Geometry check sheet. Reference: the model listing, model coordinates, mm. A direction names the side the tool comes from. Round coordinates to 2 decimals unless told otherwise and drop trailing zeros. Loops run counter-clockwise (first coordinate to the right, second up) from the corner with the lowest first, then second, coordinate; pieces in that order, holes last. Notation, with made-up numbers: (67, 32.5) -> (95, 32.5) arc R23 cw to (95, 50.5) -> close; hole circle Ø4 at (78, 25.5). An arc over 180 degrees is marked (long way). Use one line per item in the form item = value.
from build123d import *

# Parameters (mm, degrees)
SKETCH_1_R      = 1.25
EXTRUDE_1_DEPTH = 2


with BuildPart() as part:
    # 草圖1 → 填料-伸長1 (new body)
    with BuildSketch(Plane.XY):
        with BuildLine():
            Line((18.048613933, -20.404186252), (23.048613933, -20.404186252))
            ThreePointArc((23.048613933, -20.404186252), (23.755720714, -20.111293033), (24.048613933, -19.404186252))
            Line((24.048613933, -19.404186252), (24.048613933, -15.404186252))
            Line((24.048613933, -15.404186252), (24.048613933, -2.404186252))
            ThreePointArc((24.048613933, -2.404186252), (23.755720714, -1.697079471), (23.048613933, -1.404186252))
            Line((23.048613933, -1.404186252), (-6.951386067, -1.404186252))
            ThreePointArc((-6.951386067, -1.404186252), (-7.658492848, -1.697079471), (-7.951386067, -2.404186252))
            Line((-7.951386067, -2.404186252), (-7.951386067, -15.404186252))
            Line((-7.951386067, -15.404186252), (-7.951386067, -19.404186252))
            ThreePointArc((-7.951386067, -19.404186252), (-7.658492848, -20.111293033), (-6.951386067, -20.404186252))
            Line((-6.951386067, -20.404186252), (-1.951386067, -20.404186252))
            ThreePointArc((-1.951386067, -20.404186252), (-1.244279286, -20.697079471), (-0.951386067, -21.404186252))
            Line((-0.951386067, -21.404186252), (-0.951386067, -60.404186252))
            ThreePointArc((-0.951386067, -60.404186252), (8.048613933, -69.404186252), (17.048613933, -60.404186252))
            Line((17.048613933, -60.404186252), (17.048613933, -21.404186252))
            ThreePointArc((17.048613933, -21.404186252), (17.341507152, -20.697079471), (18.048613933, -20.404186252))
        make_face()
        with Locations((8.048613933, -60.404186252)):
            Circle(SKETCH_1_R, mode=Mode.SUBTRACT)
        with Locations((-5.451386067, -17.904186252)):
            Circle(SKETCH_1_R, mode=Mode.SUBTRACT)
        with Locations((21.548613933, -17.904186252)):
            Circle(SKETCH_1_R, mode=Mode.SUBTRACT)
    extrude(amount=EXTRUDE_1_DEPTH)


solid = part.part
1. Material ranges on line 1 along Y through (x, z) = (-5.5, 1); line 2 along X through (y, z) = (-45.5, 0.6); line 3 along X through (y, z) = (-61.5, 0.1), recorded low to high.
Return value:
line_1 = -20.4 to -19.15, -16.66 to -1.4
line_2 = -0.95 to 17.05
line_3 = -0.88 to 7.45, 8.65 to 16.98
2. Mould release check, pull along X, two halves, no side actions. Record for faces 1 (the cylindrical face through (-5.722, -19.124, 0.986)), 2 (the cylindrical face through (7.85, -69.4, 0.99)), 3 (the flat face through (8, -27, 2)): released by +X, released by -X, zero draft, split by the parting line, or undercut.
Return value:
face_1 = undercut
face_2 = split by the parting line
face_3 = zero draft
3. Section check B-B (x = 21.5). Record the boundary of the cut face in (y, z), then the cut area to 3 significant figures.
Return value:
outline = (-20.4, 0) -> (-19.15, 0) -> (-19.15, 2) -> (-20.4, 2) -> close; (-16.66, 0) -> (-1.4, 0) -> (-1.4, 2) -> (-16.66, 2) -> close
area = 33.0 mm2
4. Section check D-D (x = -5). Record the boundary of the cut face in (y, z).
Return value:
outline = (-20.4, 0) -> (-19.07, 0) -> (-19.07, 2) -> (-20.4, 2) -> close; (-16.74, 0) -> (-1.4, 0) -> (-1.4, 2) -> (-16.74, 2) -> close
5. Section check A-A (z = 1). Record the boundary of the cut face in (x, y), then the cut area to 3 significant figures.
Return value:
outline = (-7.95, -19.4) arc R1 ccw to (-6.95, -20.4) -> (-1.95, -20.4) arc R1 cw to (-0.95, -21.4) -> (-0.95, -60.4) arc R9 ccw to (17.05, -60.4) -> (17.05, -21.4) arc R1 cw to (18.05, -20.4) -> (23.05, -20.4) arc R1 ccw to (24.05, -19.4) -> (24.05, -2.4) arc R1 ccw to (23.05, -1.4) -> (-6.95, -1.4) arc R1 ccw to (-7.95, -2.4) -> close; hole circle Ø2.5 at (-5.45, -17.9); hole circle Ø2.5 at (8.05, -60.4); hole circle Ø2.5 at (21.55, -17.9)
area = 1,440 mm2
6. Tool access check on faces 4 (the flat face through (-0.951, -41, 1)), 5 (the flat face through (21, -20.404, 1)), 6 (the flat face through (24.049, -11, 1)). Record the directions out of +Z, -Z, +X, -X, +Y, -Y that give a thin tool (end or side, any length) a straight path to the whole face; none if there is none.
Return value:
face_4 = +Z, -Z, -X, -Y
face_5 = +Z, -Z, +X, -Y
face_6 = +Z, -Z, +X, +Y, -Y
7. Section check C-C (y = -55). Record the boundary of the cut face in (x, z), then the cut area to 3 significant figures.
Return value:
outline = (-0.95, 0) -> (17.05, 0) -> (17.05, 2) -> (-0.95, 2) -> close
area = 36.0 mm2
8. Gauge pin test, flat end, axial feed: pin 1 (1 mm diameter, centred on y = -47.5, z = 1.5, fed in from +X). Record the tip position at first contact, or that the pin passes through.
Return value:
pin_1 = 17.05
